Input: part model. Units: mm. Frame: model coordinates. A direction names the side the tool comes from. Coordinates: 2 decimals unless noted, no trailing zeros. Loops run counter-clockwise (first coordinate to the right, second up) from the corner with the lowest first, then second, coordinate; pieces in that order, holes last. Notation, with made-up numbers: M 76,63 L 104,63 A21 cw 104,81 Z; hole C -13,80 d4. An arc over 180 degrees is marked long. Use a Markdown table: item, result. Add a question column.
1. Draft query along Y for faces 1 (the flat face through (6, -1, 0)), 2 (the flat face through (-2, 1, 0)), 3 (the flat face through (-1, 0, -3)), 4 (the flat face through (-1, -2, -3)). Return one class per face: +Y half, -Y half, draft (parallel to the pull), parting line (faces both ways), or undercut.
2. Set-up query: faces 5 (the cylindrical face through (-0.645, -8.798, 4.088)), 6 (the flat face through (-7, 1, 1)), 7 (the flat face through (5, -4, 2)). Return all of +Z, -Z, +X, -X, +Y, -Y with unobstructed straight access to the full face (end or side cutting, diameter ignored); none if empty.
3. Section D-D on x = 3.75. Output: boundary loops of the cut face in (y, z).
4. Line query: L1, parallel to Y at x = -1.25, z = -1.75; L2, parallel to Z at x = -8, y = 4; L3, parallel to X at y = -3, z = 4.25. Output: solid intervals per line, ascending. Write a range as [from, to].
5. Pin query (flat end, axial travel): pin 1 (3 mm diameter, centred on x = -6.5, y = -2.5, fed in from +Z); pin 2 (1.2 mm diameter, centred on x = -2, y = 1.5, fed in from -Z); pin 3 (4.5 mm diameter, centred on x = -4.5, z = -7.5, fed in from -Y). Return the tip coordinate at first contact, or that it passes through.
6. Section C-C on z = -2. Output: boundary loops of the cut face in (x, y), then the cut area to 3 significant figures.
7. Section B-B on x = -2.25. Output: boundary loops of the cut face in (y, z).
```python
from build123d import *

# Parameters (mm, degrees)
F3_DEPTH  = 2
F4_DEPTH  = 2
F5_W      = 13
F5_H      = 4.5
F5_H_2    = 2
F6_DEPTH  = 2
F7_R      = 2
F8_DEPTH  = 11
F10_DEPTH = 3


with BuildPart() as f3:
    # F0 (on Front) → F3 (new body)
    with BuildSketch(Plane.XZ):
        with BuildLine():
            Line((0, 0), (-7, 0))
            ThreePointArc((-7, 0), (-4.9497474683, -4.9497474683), (0, -7))
            Line((0, -7), (6, -7))
            Line((6, -7), (6, 0))
            Line((6, 0), (0, 0))
        make_face()
    extrude(amount=F3_DEPTH)



with BuildPart() as f4:
    # F2 (on offset) → F4 (new body)
    with BuildSketch(Plane.XZ.offset(-2.5)):
        Polygon((6, 0), (0, 0), (-15, 0), (-15, -15), (0, -15), (6, -15), align=None)
    extrude(amount=-F4_DEPTH)


with BuildPart() as f6:
    # F5 (on face) → F6 (new body)
    with BuildSketch(Plane.XY):
        with Locations((-0.5, 2.25)):
            Rectangle(F5_W, F5_H)
        with Locations((-0.5, -1)):
            Rectangle(F5_W, F5_H_2)
    extrude(amount=F6_DEPTH)


with BuildPart() as f8:
    # F7 (on face) → F8 (new body)
    with BuildSketch(Plane.YZ.offset(6)):
        with Locations((-6.8, 4)):
            Circle(F7_R)
    extrude(amount=-F8_DEPTH)


with BuildPart() as f3_1:
    add(f3.part)

    add(f4.part)  # F10 merges F4

    add(f6.part)  # F10 merges F6

    add(f8.part)  # F10 merges F8
    # F9 (on face) → F10 (join)
    with BuildSketch(Plane.YZ.offset(6)):
        with BuildLine():
            Line((-6.8, 2), (-2, 2))
            Line((-2, 2), (-2, -7.0320754312))
            Line((-2, -7.0320754312), (4.5, -7.0320754312))
            Line((4.5, -7.0320754312), (4.5, 2))
            ThreePointArc((4.5, 2), (3.3284271247, 4.8284271247), (0.5, 6))
            Line((0.5, 6), (-6.8, 6))
            ThreePointArc((-6.8, 6), (-5.3857864376, 5.4142135624), (-4.8, 4))
            ThreePointArc((-4.8, 4), (-5.3857864376, 2.5857864376), (-6.8, 2))
        make_face()
    extrude(amount=-F10_DEPTH)


solid = f3_1.part
```
Answers below:
| question | item | result |
|---|---|---|
| 1 | face 1 | draft |
| 1 | face 2 | undercut |
| 1 | face 3 | undercut |
| 1 | face 4 | -Y half |
| 2 | face 5 | -X |
| 2 | face 6 | +Z, -X, +Y, -Y |
| 2 | face 7 | -Z, +X, -X, -Y |
| 3 | outline | M -6.8,2 L -2,2 L -2,-7.03 L 2.5,-7.03 L 2.5,-15 L 4.5,-15 L 4.5,2 A4 ccw 0.5,6 L -6.8,6 A2 ccw Z |
| 4 | L1 | y = [-2, 0], [2.5, 4.5] |
| 4 | L2 | z = [-15, 0] |
| 4 | L3 | x = [3, 6] |
| 5 | pin 1 | stops at z = 2 |
| 5 | pin 2 | stops at z = 0 |
| 5 | pin 3 | stops at y = -2 |
| 6 | outline | M -15,2.5 L 3,2.5 L 3,0 L -6.71,0 L -6.71,-2 L 6,-2 L 6,4.5 L -15,4.5 Z |
| 6 | area | 74.9 mm² |
| 7 | outline | C -6.8,4 d4; M -2,-6.63 L 0,-6.63 L 0,0 L 2.5,0 L 2.5,-15 L 4.5,-15 L 4.5,2 L -2,2 Z |
